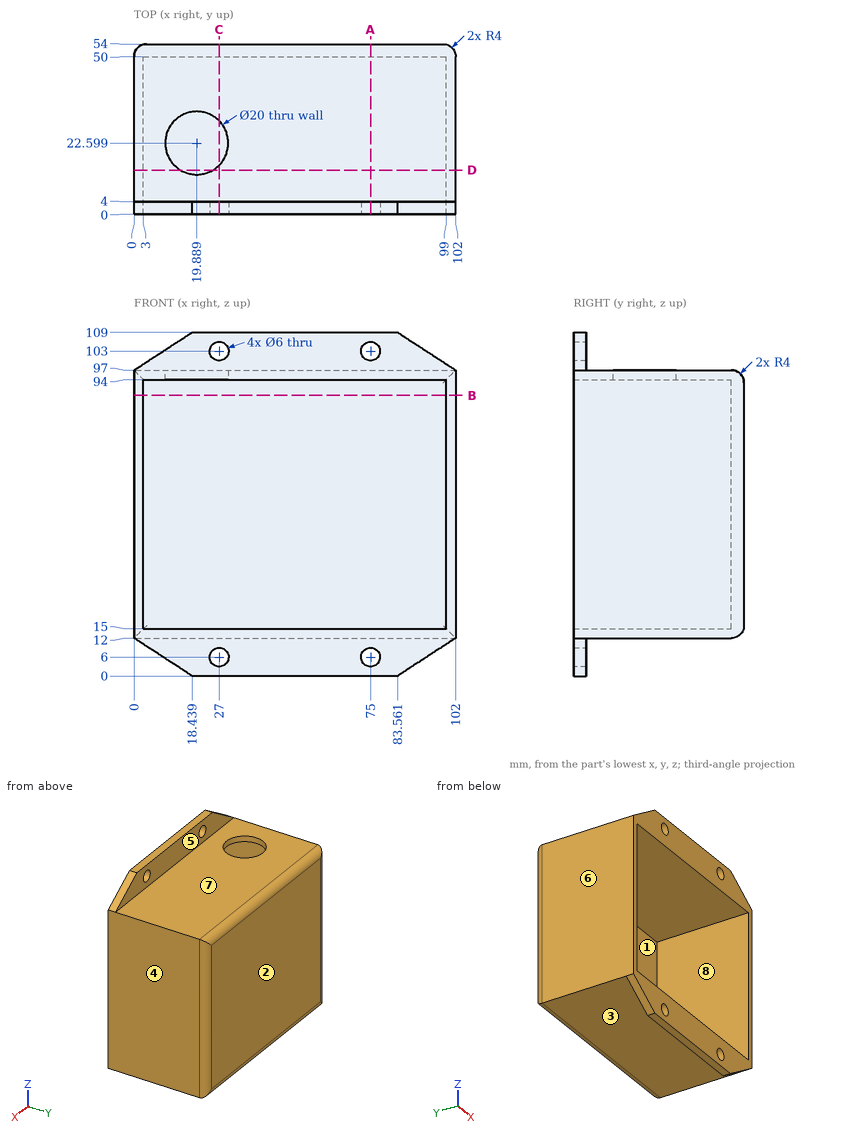
Part print with two shaded views. Sizes in mm from the minimum x, y, z corner. A direction names the side the tool comes from. Coordinates: 2 decimals unless noted, no trailing zeros. Write each loop counter-clockwise with the first axis right and the second up, starting at its lowest first coordinate (ties: lowest second). Pieces come first, ordered by that corner, then holes. Notation, with made-up numbers: M 67.5,31 L 93.5,31 A10 ccw 93.5,42 Z; hole C 12.25,64 d9. An arc over 180 degrees is marked long. Return JSON: item names as keys, results as strings.
Item 1: Probe line 1 (Z direction, x = 13.5, y = 43); line 2 (X direction, y = 25.5, z = 93.5); line 3 (X direction, y = 1.6, z = 103). List the from-to ranges inside material, lowest first. Write a range as from..to.
Findings below:
{"line 1": "z = 12..15, 94..97", "line 2": "x = 0..3, 99..102", "line 3": "x = 9.22..24, 30..72, 78..92.78"}
Item 2: Drop flat-ended pins along their axis: pin 1 Ø9.5 at (x, z) = (34.5, 102) entering from +Y; pin 2 Ø18 at (x, y) = (19.89, 22.6) entering from -Z; pin 3 Ø2 at (x, z) = (46.5, 39.5) entering from -Y; pin 4 Ø9.5 at (x, z) = (27, 103) entering from -Y. Give the stop position or say it passes through.
Findings below:
{"pin 1": "stops at y = 4", "pin 2": "stops at z = 12", "pin 3": "stops at y = 50", "pin 4": "stops at y = 0"}
Item 3: Slice it at B-B, the plane z = 89. Write the cut outline in (x, y).
Findings below:
{"outline": "M 0,0 L 3,0 L 3,50 L 99,50 L 99,0 L 102,0 L 102,50 A4 ccw 98,54 L 4,54 A4 ccw 0,50 Z"}
Item 4: Slice it at A-A, the plane x = 75. Write the cut outline in (y, z), and give its area (3 significant figures).
Findings below:
{"outline": "M 0,0 L 4,0 L 4,3 L 0,3 Z; M 0,9 L 4,9 L 4,12 L 50,12 A4 ccw 54,16 L 54,93 A4 ccw 50,97 L 4,97 L 4,100 L 0,100 L 0,94 L 50,94 L 50,15 L 0,15 Z; M 0,106 L 4,106 L 4,109 L 0,109 Z", "area": "681 mm2"}
Item 5: Slice it at C-C, the plane x = 27. Write the cut outline in (y, z).
Findings below:
{"outline": "M 0,0 L 4,0 L 4,3 L 0,3 Z; M 0,9 L 4,9 L 4,12 L 50,12 A4 ccw 54,16 L 54,93 A4 ccw 50,97 L 29.63,97 L 29.63,94 L 50,94 L 50,15 L 0,15 Z; M 0,94 L 15.57,94 L 15.57,97 L 4,97 L 4,100 L 0,100 Z; M 0,106 L 4,106 L 4,109 L 0,109 Z"}
Item 6: Which spindle directions (+Z, -Z, +X, -X, +Y, -Y) get a long thin tool onto all of the face, cutting with end or side? Do the marked faces 1, 2, 3, 4 and 5. Say none if no direction does.
Findings below:
{"face 1": "-Y", "face 2": "+Z, -Z, +X, -X, +Y", "face 3": "-Z, +X, -X, +Y", "face 4": "+Z, -Z, +X, +Y, -Y", "face 5": "+Z, +X, -X, +Y"}
Item 7: Slice it at D-D, the plane y = 14. Write the cut outline in (x, z), and give its area (3 significant figures).
Findings below:
{"outline": "M 0,12 L 102,12 L 102,97 L 24.99,97 L 24.99,94 L 99,94 L 99,15 L 3,15 L 3,94 L 14.78,94 L 14.78,97 L 0,97 Z", "area": "1,060 mm2"}
Item 8: Two-plate mould, pull along Z, no slides. Class the marked faces 6, 7 and 8: +Z half, -Z half, draft (parallel to the pull), parting line (faces both ways), or undercut.
Findings below:
{"face 6": "draft", "face 7": "+Z half", "face 8": "undercut"}
